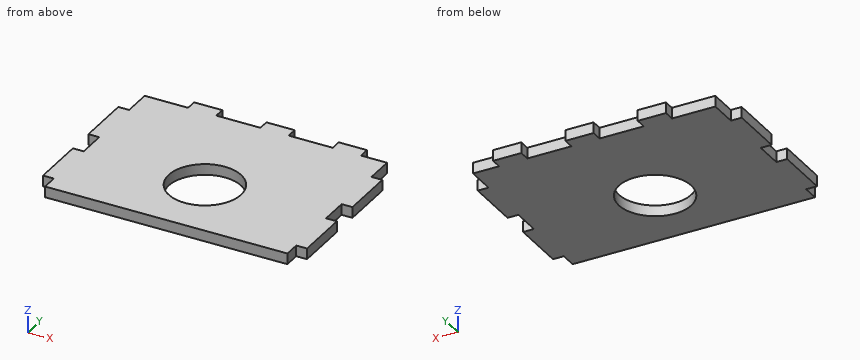
from build123d import *

# Parameters (mm, degrees)
SKETCH1_W           = 73
SKETCH1_H           = 50
BOSS_EXTRUDE1_DEPTH = 3
SKETCH2_W           = 3
SKETCH2_H           = 7.8
CUT_EXTRUDE1_DEPTH  = 53.999062732
LPATTERN1_COUNT     = 3
LPATTERN1_PITCH     = 22.8
SKETCH3_W           = 3
SKETCH3_H           = 7.8
CUT_EXTRUDE2_DEPTH  = 53.999062732
LPATTERN2_COUNT     = 4
LPATTERN2_PITCH     = 22.8
SKETCH6_W           = 3
SKETCH6_H           = 19.4
CUT_EXTRUDE3_DEPTH  = 10
SKETCH7_W           = 7.8
SKETCH7_H           = 3
BOSS_EXTRUDE2_DEPTH = 3
LPATTERN3_COUNT     = 3
LPATTERN3_PITCH     = 20
SKETCH8_W           = 3
SKETCH8_H           = 15
BOSS_EXTRUDE3_DEPTH = 3
CUT_EXTRUDE4_REACH  = 54.999
SKETCH9_R           = 10


with BuildPart() as part:
    # Sketch1 → Boss-Extrude1 (new body)
    with BuildSketch(Plane.XY):
        with Locations((-4.493460648, -8.457986111)):
            Rectangle(SKETCH1_W, SKETCH1_H)
    extrude(amount=BOSS_EXTRUDE1_DEPTH)

    # Sketch2 → Cut-Extrude1 (cut, through all)
    with BuildSketch(Plane.XY.offset(3)):
        with Locations((-39.493460648, 12.642013889)):
            Rectangle(SKETCH2_W, SKETCH2_H)
    cut_extrude1 = extrude(amount=-CUT_EXTRUDE1_DEPTH, mode=Mode.SUBTRACT)

    # LPattern1: Cut-Extrude1 ×3
    with Locations(*[(0, -i * LPATTERN1_PITCH, 0) for i in range(1, LPATTERN1_COUNT)]):
        add(cut_extrude1, mode=Mode.SUBTRACT)

    # Sketch3 → Cut-Extrude2 (cut, through all)
    with BuildSketch(Plane.XY.offset(3)):
        with Locations((30.506539352, 12.642013889)):
            Rectangle(SKETCH3_W, SKETCH3_H)
    cut_extrude2 = extrude(amount=-CUT_EXTRUDE2_DEPTH, mode=Mode.SUBTRACT)

    # LPattern2: Cut-Extrude2 ×4
    with Locations(*[(0, -i * LPATTERN2_PITCH, 0) for i in range(1, LPATTERN2_COUNT)]):
        add(cut_extrude2, mode=Mode.SUBTRACT)

    # Sketch6 → Cut-Extrude3 (cut)
    with BuildSketch(Plane.XY.offset(3)):
        with Locations((-39.493460648, -23.757986111)):
            Rectangle(SKETCH6_W, SKETCH6_H)
    extrude(amount=-CUT_EXTRUDE3_DEPTH, mode=Mode.SUBTRACT)

    # Sketch7 → Boss-Extrude2 (add)
    with BuildSketch(Plane(origin=(0, 16.542013889, 0), x_dir=(1, 0, 0), z_dir=(0, 1, 0))):
        with Locations((-22.093460648, -1.5)):
            Rectangle(SKETCH7_W, SKETCH7_H)
    boss_extrude2 = extrude(amount=BOSS_EXTRUDE2_DEPTH)

    # LPattern3: Boss-Extrude2 ×3
    with Locations(*[(i * LPATTERN3_PITCH, 0, 0) for i in range(1, LPATTERN3_COUNT)]):
        add(boss_extrude2)

    # Sketch8 → Boss-Extrude3 (add)
    with BuildSketch(Plane.ZY.offset(37.993460648)):
        with Locations((1.5, -21.557986111)):
            Rectangle(SKETCH8_W, SKETCH8_H)
    extrude(amount=BOSS_EXTRUDE3_DEPTH)

    # Sketch9 → Cut-Extrude4 (cut, up to next)
    with BuildSketch(Plane.XY.offset(3), mode=Mode.PRIVATE) as cut_extrude4_sk1:
        with Locations((-4.493460648, -14.057986111)):
            Circle(SKETCH9_R)
    cut_extrude4_tool1 = extrude(cut_extrude4_sk1.sketch, amount=-CUT_EXTRUDE4_REACH, mode=Mode.PRIVATE) & part.part
    add(cut_extrude4_tool1.solids().sort_by_distance((-4.493461, -14.057986, 3))[0], mode=Mode.SUBTRACT)


solid = part.part
Can you work these out from the model? Positions are in its coordinate system, mm. Give positions to 0.01 mm unless a question says otherwise; leave off trailing zeros. Order: outer loops, then holes, each group sorted by start corner. A loop starts at its lowest first (then second) coordinate and runs counter-clockwise, first axis right, second up. Notation, with made-up numbers: M -22,-37.75 L 26,-37.75 A6 cw 26,-32.75 Z; hole C -3.75,-7 d5. An arc over 180 degrees is marked long. Use a Markdown table: item, result. Add a question column.
Item 1: Will these pins go through, and if not, where does the flat tip stop? pin 1 (0.9 mm diameter, centred on x = 27, z = 2, fed in from +Y); pin 2 (8 mm diameter, centred on x = -20, y = -6.5, fed in from -Z); pin 3 (1.5 mm diameter, centred on y = 18, z = 1, fed in from -X); pin 4 (0.9 mm diameter, centred on x = 30.5, z = 1, fed in from +Y).
Item 2: Suppose I cut it at C-C (x = -7.5). List the corners of the cut face in (y, z) for me.
Item 3: If I drill on L1, parallel to Y at x = -16.5, z = 2.75; L2, parallel to Y at x = -5, z = 0.45; L3, parallel to X at y = -19.5, z = 1, over which ranges is the centre line in solid material (lowest first)? Write a range as [from, to].
Item 4: Suppose I cut it at B-B (y = -21.5). List the corners of the cut face in (x, z) for me.
Item 5: Suppose I cut it at D-D (x = 27). List the corners of the cut face in (y, z) for me, then the cut area to 3 significant figures.
Answer sheet:
| question | item | result |
|---|---|---|
| 1 | pin 1 | stops at y = 16.54 |
| 1 | pin 2 | stops at z = 0 |
| 1 | pin 3 | stops at x = -25.99 |
| 1 | pin 4 | stops at y = 8.74 |
| 2 | outline | M -33.46,0 L -23.6,0 L -23.6,3 L -33.46,3 Z; M -4.52,0 L 16.54,0 L 16.54,3 L -4.52,3 Z |
| 3 | L1 | y = [-33.46, 16.54] |
| 3 | L2 | y = [-33.46, -24.05], [-4.07, 19.54] |
| 3 | L3 | x = [-40.99, -12.88], [3.9, 32.01] |
| 4 | outline | M -40.99,0 L -11.17,0 L -11.17,3 L -40.99,3 Z; M 2.19,0 L 32.01,0 L 32.01,3 L 2.19,3 Z |
| 5 | outline | M -33.46,0 L 16.54,0 L 16.54,3 L -33.46,3 Z |
| 5 | area | 150 mm² |
